Autodesk Inventor part; units mm, degrees
ref_plane "YZ Plane" through (0, 0, 0) normal (1, 0, 0) x (0, 1, 0)
ref_plane "XZ Plane" through (0, 0, 0) normal (0, 1, 0) x (-1, 0, 0)
ref_plane "XY Plane" through (0, 0, 0) normal (0, 0, 1) x (1, 0, 0)
sketch "Sketch1" plane through (0, 0, 0) normal (0, 1, 0) x (-1, 0, 0)
  line L0 (6.25, 5.75) -> (-6.25, 5.75)
  line L1 (-6.25, 5.75) -> (-6.25, -5.75)
  line L2 (-6.25, -5.75) -> (6.25, -5.75)
  line L3 (6.25, -5.75) -> (6.25, 5.75)
  line L4 (6.25, 5.75) -> (-6.25, -5.75) construction
  line L5 (-6.25, 5.75) -> (6.25, -5.75) construction
  point P0 (0, 0)
  dimension "d0" = 12.5
  dimension "d1" = 11.5
extrude "Extrusion1" add sketch "Sketch1" along normal blind 7.5
sketch "Sketch2" plane through (0, 7.5, 0) normal (0, 1, 0) x (1, 0, 0)
  circle A0 centre (0, 0) radius 3.75
  dimension "d4" = 7.5
extrude "Extrusion2" add sketch "Sketch2" along normal blind 7
sketch "Sketch3" plane through (0, 14.5, 0) normal (0, 1, 0) x (1, 0, 0)
  circle A0 centre (0, 0) radius 3
  dimension "d7" = 6
extrude "Extrusion3" add sketch "Sketch3" along normal blind 13
sketch "Sketch4" plane through (0, 27.5, 0) normal (0, 1, 0) x (1, 0, 0)
  circle A0 centre (0, 0) radius 3
  line L0 (1.5, -2.5981) -> (1.5, 2.5981)
  line L1 (3, 0) -> (-9, 0) construction
  circle A1 centre (0, 0) radius 3.75 construction
  circle A2 centre (0, 0) radius 3 construction
  point P0 (-3, 0)
  dimension "d10" = 4.5
extrude "Extrusion4" cut sketch "Sketch4" against normal blind 10 contours A0 L0 picked at (1.6691, 0.7431)
chamfer "Chamfer1" distance 0.5 angle 45 1 edges at (-3.75, 14.5, 0)
chamfer "Chamfer2" distance 1 angle 45 1 edges at (-3, 27.5, 0)
properties part number "rotery"
For this review, take the finished solid that the model builds, in its own axes (mm). A direction names the side the tool comes from. Round coordinates to 2 decimals unless told otherwise and drop trailing zeros. Write each loop counter-clockwise with the first axis right and the second up, starting at its lowest first coordinate (ties: lowest second). Pieces come first, ordered by that corner, then holes. Notation, with made-up numbers: M 67,1.25 L 115,1.25 A25 cw 115,27.25 Z; hole C 29,-30.5 d9. An arc over 180 degrees is marked long. Write item = value, one per line. Start each with the question number.
(1) We need section C-C (y = 8.75). Give the boundary of the cut face in (x, z), then the cut area to 3 significant figures.
(2) We need section B-B (z = 0). Give the boundary of the cut face in (x, y).
(3) For line 1 along Y through (x, z) = (5, -4.25); line 2 along Z through (x, y) = (-1.5, 22); line 3 along X through (y, z) = (11, 0), list the stretches that pass through material, from the lowest coordinate up.
(4) We need section A-A (x = 0). Give the boundary of the cut face in (y, z), then the cut area to 4 significant figures.
(5) Clearance check with flat-ended pins moving along their axes: pin 1 Ø1.2 at (x, z) = (2, -0.5) entering from +Y; pin 2 Ø1 at (x, y) = (-2, 15.5) entering from +Z; pin 3 Ø1.5 at (x, y) = (4, 9) entering from -Z; pin 4 Ø1.5 at (x, y) = (-1.5, 20) entering from -Z. State where each tip first meets the part, or that it passes through.
(6) For faces 1 (the face through (0, 4, -5.75)), 2 (the face through (2, 17.5, 0)), 3 (the face through (-2.4, 20.4, -1.8)), list the 3-axis set-ups (+Z, -Z, +X, -X, +Y, -Y) from which the entire face can be reached by the end or side of a thin tool; tool diameter is ignored.
(7) We need section D-D (x = 5). Give the boundary of the cut face in (y, z), then the cut area to 4 significant figures.
Results found:
q1.outline = C 0,0 d7.5
q1.area = 44.2 mm²
q2.outline = M -6.25,0 L 6.25,0 L 6.25,7.5 L 3.75,7.5 L 3.75,14 L 3.25,14.5 L 3,14.5 L 3,17.5 L 1.5,17.5 L 1.5,27.5 L -2,27.5 L -3,26.5 L -3,14.5 L -3.25,14.5 L -3.75,14 L -3.75,7.5 L -6.25,7.5 Z
q3.line_1 = 0 to 7.5
q3.line_2 = -2.6 to 2.6
q3.line_3 = -3.75 to 3.75
q4.outline = M 0,-5.75 L 7.5,-5.75 L 7.5,-3.75 L 14,-3.75 L 14.5,-3.25 L 14.5,-3 L 26.5,-3 L 27.5,-2 L 27.5,2 L 26.5,3 L 14.5,3 L 14.5,3.25 L 14,3.75 L 7.5,3.75 L 7.5,5.75 L 0,5.75 Z
q4.area = 215.5 mm²
q5.pin_1 = 27.5
q5.pin_2 = 2.6
q5.pin_3 = -1.87
q5.pin_4 = -2.9
q6.face_1 = -Z, +X, -X, +Y, -Y
q6.face_2 = +Z, -Z, +X, +Y
q6.face_3 = +Y
q7.outline = M 0,-5.75 L 7.5,-5.75 L 7.5,5.75 L 0,5.75 Z
q7.area = 86.25 mm²
